Geometry check sheet. Reference: the model listing, model coordinates, mm. Round coordinates to 2 decimals unless told otherwise and drop trailing zeros. Order: outer loops, then holes, each group sorted by start corner. A loop starts at its lowest first (then second) coordinate and runs counter-clockwise, first axis right, second up.
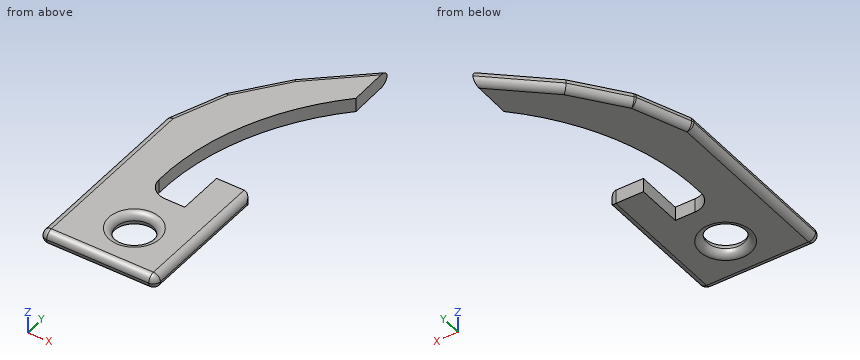
```python
from build123d import *

# Parameters (mm, degrees)
F0_R     = 5.08
F1_DEPTH = 3.81
F2_R     = 1.90499
F4_R     = 5.08


# Not quite as in the source:
# - two fillets or chamfers of one size are made in one step
# - a fillet or chamfer is up to 0.001 mm smaller than in the source, because OpenCascade refuses the exact size


with BuildPart() as f1:
    # F0 (on Top) → F1 (new body)
    with BuildSketch(Plane.XY):
        with BuildLine():
            Line((-5.6879511814, 25.4), (-5.6879511814, -25.4))
            Line((-5.6879511814, -25.4), (5.6879511814, -25.4))
            Line((5.6879511814, -25.4), (26.0620488186, -25.4))
            Line((26.0620488186, -25.4), (26.0620488186, 0))
            Line((26.0620488186, 0), (26.0620488186, 12.7))
            Line((26.0620488186, 12.7), (16.6040229345, 12.7))
            Line((16.6040229345, 12.7), (16.6040229345, 0))
            Line((16.6040229345, 0), (6.4440229345, 0))
            ThreePointArc((6.4440229345, 0), (10.1083489192, 29.4811569654), (26.0620488186, 54.5419901609))
            Line((26.0620488186, 54.5419901609), (25.8431795214, 67.2401040457))
            Line((25.8431795214, 67.2401040457), (10.0171072409, 53.1962551177))
            Line((10.0171072409, 53.1962551177), (0, 40.1331372559))
            Line((0, 40.1331372559), (-5.6879511814, 25.4))
        make_face()
        with Locations((11.5240229345, -12.7)):
            Circle(F0_R, mode=Mode.SUBTRACT)
    extrude(amount=F1_DEPTH)

    # F2 (radius 1.905 in the source; OpenCascade refuses exactly that, so slightly less here)
    f2_edges = [f1.edges().sort_by_distance(p)[0] for p in [
        (-5.687951, 0, 3.81),
        (10.187049, -25.4, 3.81),
        (10.187049, -25.4, 0),
        (26.062049, -6.35, 3.81),
        (26.062049, -6.35, 0),
        (26.062049, -25.4, 1.905),
        (-5.687951, -25.4, 1.905),
        (26.062049, 12.7, 1.905),
        (-2.843976, 32.766569, 3.81),
        (-2.843976, 32.766569, 0),
        (-5.687951, 0, 0),
        (6.444023, -12.7, 0),
        (6.444023, -12.7, 3.81),
        (17.930143, 60.21818, 0),
        (17.930143, 60.21818, 3.81),
        (5.008554, 46.664696, 3.81),
        (-5.687951, 25.4, 1.905),
        (0, 40.133137, 1.905),
        (5.008554, 46.664696, 0),
    ]]
    fillet(f2_edges, radius=F2_R)

    # F4
    f4_edges = [f1.edges().sort_by_distance(p)[0] for p in [
        (6.444023, 0, 1.905),
    ]]
    fillet(f4_edges, radius=F4_R)


solid = f1.part
```
(1) Depth check by flat-ended pin: P1, Ø12, axis at x = 14, y = 36.5, coming from the +Z side; P2, Ø1.9, axis at x = 13.5, z = 1.5, coming from the +Y side; P3, Ø2, axis at y = 12.5, z = 0.5, coming from the -X side; P4, Ø1, axis at x = 0, z = 2.5, coming from the +Y side. Enter the tip coordinate at first touch or a pass-through.
Returned:
P1: stops at z = 3.81
P2: stops at y = 57.1
P3: stops at x = -5.64
P4: stops at y = 40.67
(2) Material ranges on line 1 (Y direction, x = 12, z = 2.9); line 2 (X direction, y = -12.7, z = 1.9); line 3 (Y direction, x = 16, z = 2.95), recorded low to high.
Returned:
line 1: y = -25.12 to -18.04, -7.36 to 0, 34.18 to 54.58
line 2: x = -5.69 to 6.44, 16.6 to 26.06
line 3: y = -25.09 to -15.71, -9.69 to 0, 41.79 to 58.09
(3) Sectioned sample at B-B, the plane z = 0.85. Record the cut outline in (x, y) (3 decimals).
Returned:
outline: (-5.369, -23.495) arc R1.586 ccw to (-3.783, -25.081) - (24.157, -25.081) arc R1.586 ccw to (25.743, -23.495) - (25.743, 11.85) arc R1.905 ccw to (24.157, 12.7) - (16.604, 12.7) - (16.604, 0) - (11.219, 0) arc R5.08 cw to (6.14, 4.956) arc R67.577 cw to (26.062, 54.542) - (25.85, 66.82) - (10.252, 52.978) - (0.42, 40.157) arc R1.586 ccw to (0.199, 39.763) - (-5.263, 25.616) arc R1.586 ccw to (-5.369, 25.045) - close; hole circle Ø10.798 at (11.524, -12.7)
(4) Sectioned sample at C-C, the plane x = 8.5. Give the number of separate pieces and of enclosed holes in the cut face, and give its area (3 significant figures).
Returned:
separate pieces: 3
enclosed holes: 0
area: 163 mm2
